Check sheet for the drawn part. Datum: minimum x, y, z corner. Units: mm. Give positions to 0.01 mm unless a question says otherwise; leave off trailing zeros. Loops run counter-clockwise (first coordinate to the right, second up) from the corner with the lowest first, then second, coordinate; pieces in that order, holes last. Notation, with made-up numbers: (-3.5, 28.25) - (53.5, 28.25) arc R38 cw to (53.5, 67.25) - close; hole circle Ø4 at (30, 12). An arc over 180 degrees is marked (long way). Use a Markdown table: item, result. Add a question column.
1. Material ranges on L1, parallel to X at y = 33.5, z = 1.95 (1 decimal); L2, parallel to X at y = 38.5, z = 1 (1 decimal); L3, parallel to Y at x = 29, z = 2.7, recorded low to high.
2. Cross-section at A-A on y = 33. Enter the section's corners in (x, z).
3. Cross-section at D-D on z = 2.4. Count the separate pieces of the cut face and the enclosed holes in it, and give its area (3 significant figures).
4. Cross-section at C-C on y = 58. Enter the section's corners in (x, z).
5. Depth check by flat-ended pin: P1, Ø3.5, axis at x = 20.63, y = 45.37, coming from the -Z side; P2, Ø1.5, axis at y = 13.5, z = 1, coming from the +X side (1 decimal). Enter the tip coordinate at first touch or a pass-through.
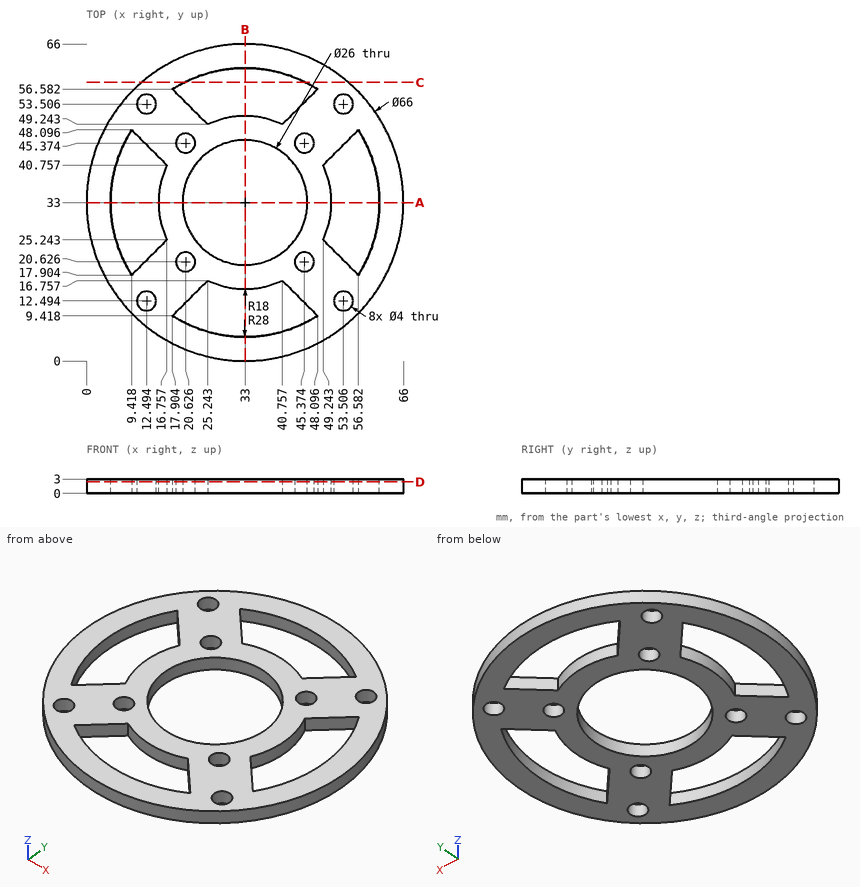
Values found:
| question | item | result |
|---|---|---|
| 1 | L1 | x = 0 to 5, 15 to 20, 46 to 51, 61 to 66 |
| 1 | L2 | x = 0.5 to 5.5, 15.9 to 21.2, 44.8 to 50.1, 60.5 to 65.5 |
| 1 | L3 | y = 0.24 to 5.29, 15.45 to 20.63, 45.37 to 50.55, 60.71 to 65.76 |
| 2 | outline | (0, 0) - (5, 0) - (5, 3) - (0, 3) - close; (15, 0) - (20, 0) - (20, 3) - (15, 3) - close; (46, 0) - (51, 0) - (51, 3) - (46, 3) - close; (61, 0) - (66, 0) - (66, 3) - (61, 3) - close |
| 3 | separate pieces | 1 |
| 3 | enclosed holes | 13 |
| 3 | area | 1,830 mm2 |
| 4 | outline | (11.46, 0) - (20.39, 0) - (20.39, 3) - (11.46, 3) - close; (45.61, 0) - (54.54, 0) - (54.54, 3) - (45.61, 3) - close |
| 5 | P1 | passes through |
| 5 | P2 | stops at x = 60.2 |
